```python
from build123d import *

# Parameters (mm, degrees)
EXTRUDE_1_DEPTH     = 60
SKETCH_2_R          = 2.75
CUT_EXTRUDE_1_DEPTH = 109.282039139
SKETCH_3_R          = 10
SKETCH_3_R_2        = 1.65
CUT_EXTRUDE_2_DEPTH = 109.282039139
CHAMFER_1_SIZE      = 5


with BuildPart() as part:
    # 草图1 → 凸台-拉伸1 (new body)
    with BuildSketch(Plane.XY):
        Polygon((0, 0), (-45, 0), (-45, 30), (-85, 30), (-85, 35), (-40, 35), (-40, 5), (0, 5), align=None)
    extrude(amount=EXTRUDE_1_DEPTH)

    # 草图2 → 切除-拉伸1 (cut, through all)
    with BuildSketch(Plane.XZ.offset(-30)):
        with Locations((-55, 50)):
            Circle(SKETCH_2_R)
        with Locations((-55, 30)):
            Circle(SKETCH_2_R)
        with Locations((-75, 30)):
            Circle(SKETCH_2_R)
        with Locations(Location((-55, 10, 0), (0, 0, 180))):
            Circle(SKETCH_2_R)
        with Locations((-75, 50)):
            Circle(SKETCH_2_R)
        with Locations((-75, 10)):
            Circle(SKETCH_2_R)
    extrude(amount=-CUT_EXTRUDE_1_DEPTH, mode=Mode.SUBTRACT)

    # 草图3 → 切除-拉伸2 (cut, through all)
    with BuildSketch(Plane(origin=(0, 5, 0), x_dir=(1, 0, 0), z_dir=(0, 1, 0))):
        with Locations(Location((-20, -30, 0), (0, 0, 180))):
            Circle(SKETCH_3_R)
        with Locations(Location((-20, -15.5, 0), (0, 0, 180))):
            Circle(SKETCH_3_R_2)
        with Locations(Location((-20, -44.5, 0), (0, 0, 180))):
            Circle(SKETCH_3_R_2)
    extrude(amount=-CUT_EXTRUDE_2_DEPTH, mode=Mode.SUBTRACT)

    # 倒角1
    chamfer_1_edges = [part.edges().sort_by_distance(p)[0] for p in [
        (-40, 5, 30),
    ]]
    chamfer(chamfer_1_edges, length=CHAMFER_1_SIZE)


solid = part.part
```
The model under review builds one solid part; all positions refer to its coordinate system, in mm. A direction names the side the tool comes from. Coordinates: 2 decimals unless noted, no trailing zeros. Write each loop counter-clockwise with the first axis right and the second up, starting at its lowest first coordinate (ties: lowest second). Pieces come first, ordered by that corner, then holes. Notation, with made-up numbers: (41.25, 84.5) - (46.25, 84.5) arc R9 ccw to (46.25, 100.5) - close; hole circle Ø1 at (1.25, 63). An arc over 180 degrees is marked (long way). Write item = value, one per line.
(1) Consider section A-A, the plane x = -20. Give the boundary of the cut face in (y, z).
Result sheet:
outline = (0, 0) - (5, 0) - (5, 13.85) - (0, 13.85) - close; (0, 17.15) - (5, 17.15) - (5, 20) - (0, 20) - close; (0, 40) - (5, 40) - (5, 42.85) - (0, 42.85) - close; (0, 46.15) - (5, 46.15) - (5, 60) - (0, 60) - close
(2) For P1, Ø4.5, axis at x = -20, z = 44.5, coming from the -Y side; P2, Ø7.5, axis at y = 17.5, z = 37, coming from the +X side; P3, Ø3.5, axis at x = -75, z = 10, coming from the -Y side; P4, Ø6.5, axis at x = -55, z = 30, coming from the -Y side, all flat-tipped, find the tip position at first contact; note any pin that passes through.
Result sheet:
P1 = 0
P2 = -40
P3 = through
P4 = 30
(3) Consider section B-B, the plane z = 30. Give the boundary of the cut face in (x, y).
Result sheet:
outline = (-85, 30) - (-77.75, 30) - (-77.75, 35) - (-85, 35) - close; (-72.25, 30) - (-57.75, 30) - (-57.75, 35) - (-72.25, 35) - close; (-52.25, 30) - (-45, 30) - (-45, 0) - (-30, 0) - (-30, 5) - (-35, 5) - (-40, 10) - (-40, 35) - (-52.25, 35) - close; (-10, 0) - (0, 0) - (0, 5) - (-10, 5) - close
(4) Machinability: for faces 4 (the face through (-45, 15, 30)), 5 (the face through (-10, 5, 36)), 6 (the face through (-24.614, 2.535, 21.128)), which of the approach directions +Z, -Z, +X, -X, +Y, -Y give a long, thin tool a straight path to every point of the face, cutting with its end or side? Answer none if there is none.
Result sheet:
face_4 = +Z, -Z, -X, -Y
face_5 = +Z, -Z, +X, +Y
face_6 = +Y, -Y
(5) Consider section C-C, the plane z = 15.5. Give the boundary of the cut face in (x, y).
Result sheet:
outline = (-85, 30) - (-45, 30) - (-45, 0) - (-21.65, 0) - (-21.65, 5) - (-35, 5) - (-40, 10) - (-40, 35) - (-85, 35) - close; (-18.35, 0) - (0, 0) - (0, 5) - (-18.35, 5) - close
(6) Mouldability with a two-part tool opening along Z and no side actions: class faces 1 (the face through (-42, 18, 0)), 2 (the face through (-32, 0, 30)), 3 (the face through (-18.69, 2.54, 14.5)) as pulls with the +Z half, pulls with the -Z half, needs draft (parallel to the pull), parting line crosses it, or undercut.
Result sheet:
face_1 = pulls with the -Z half
face_2 = needs draft
face_3 = undercut
(7) Consider section D-D, the plane x = -75. Give the boundary of the cut face in (y, z).
Result sheet:
outline = (30, 0) - (35, 0) - (35, 7.25) - (30, 7.25) - close; (30, 12.75) - (35, 12.75) - (35, 27.25) - (30, 27.25) - close; (30, 32.75) - (35, 32.75) - (35, 47.25) - (30, 47.25) - close; (30, 52.75) - (35, 52.75) - (35, 60) - (30, 60) - close
(8) For line 1 (Z direction, x = -75, y = 32); line 2 (X direction, y = 27.5, z = 5.5); line 3 (Y direction, x = -14.5, z = 38.5), list the stretches that pass through material, from the lowest coordinate up. Write a range as [from, to].
Result sheet:
line_1 = [0, 7.25], [12.75, 27.25], [32.75, 47.25], [52.75, 60]
line_2 = [-45, -40]
line_3 = [0, 5]
